Design review of the part shown in the three views and the two pictorial views. Dimensions are in mm from the part's minimum x, y and z. Give positions to 0.01 mm unless a question says otherwise; leave off trailing zeros. Loops run counter-clockwise (first coordinate to the right, second up) from the corner with the lowest first, then second, coordinate; pieces in that order, holes last. Notation, with made-up numbers: (25.5, -15) - (67.5, -15) arc R5 cw to (67.5, -9) - close; hole circle Ø10 at (-4.5, -11.75). An arc over 180 degrees is marked (long way). Use CSV: the item, a comma, the result in double quotes. Start each with the question number.
1. Take a section at C-C on z = 24.5. Give the boundary of the cut face in (x, y), plus the area to 3 significant figures.
2. Mouldability with a two-part tool opening along Y and no side actions: class the marked faces 1, 2 and 3 as pulls with the +Y half, pulls with the -Y half, needs draft (parallel to the pull), parting line crosses it, or undercut.
3. Take a section at D-D on x = 93. Give the boundary of the cut face in (y, z), plus the area to 3 significant figures.
4. Wall thickness on line 1 (Y direction, x = 10, z = 4.25); line 2 (Y direction, x = 75, z = 16.5); line 3 (Z direction, x = 90, y = 7.5): over which ranges is each line inside the solid? List them lowest first.
5. Take a section at B-B on x = 75. Give the boundary of the cut face in (y, z), plus the area to 3 significant figures.
6. Take a section at A-A on x = 140. Give the boundary of the cut face in (y, z).
7. For pin 1 (6 mm diameter, centred on y = 20, z = 22.5, fed in from +X); pin 2 (5 mm diameter, centred on x = 130, y = 14, fed in from +Z); pin 3 (4 mm diameter, centred on y = 12.5, z = 41.5, fed in from +X); pin 4 (5 mm diameter, centred on x = 38.5, y = 11.5, fed in from -Z), all flat-tipped, find the tip position at first contact; note any pin that passes through.
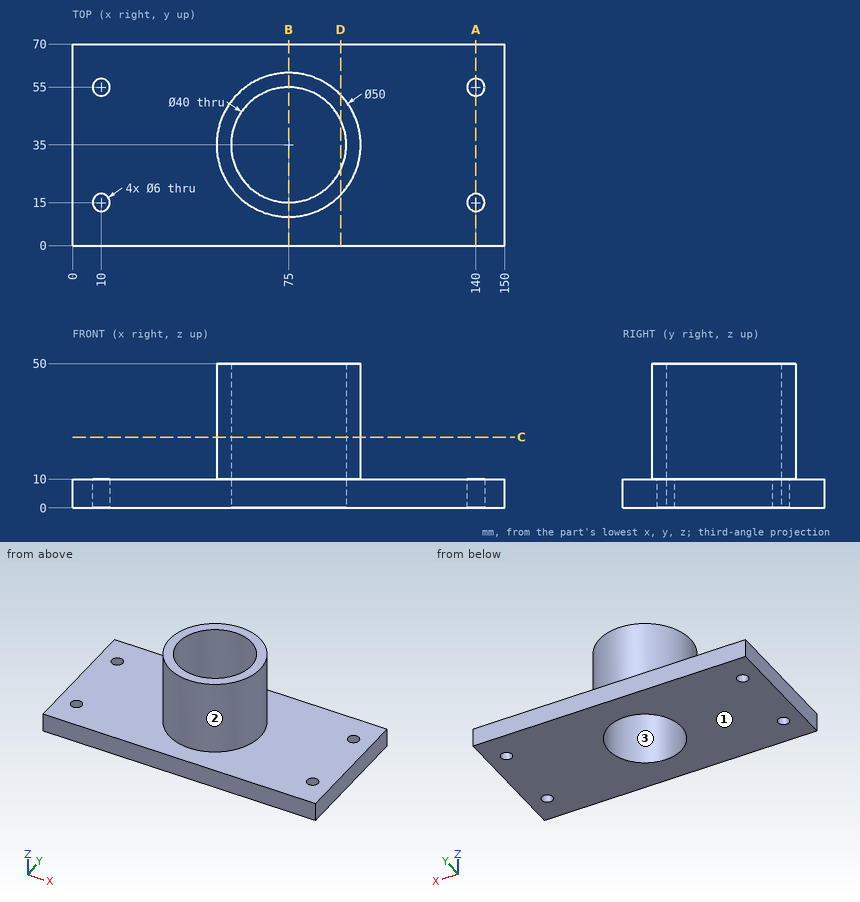
Check result:
1,outline,"circle Ø50 at (75, 35); hole circle Ø40 at (75, 35)"
1,area,"707 mm²"
2,face 1,"needs draft"
2,face 2,"parting line crosses it"
2,face 3,"undercut"
3,outline,"(0, 0) - (26.28, 0) - (26.28, 50) - (17.65, 50) - (17.65, 10) - (0, 10) - close; (43.72, 0) - (70, 0) - (70, 10) - (52.35, 10) - (52.35, 50) - (43.72, 50) - close"
3,area,"1,220 mm²"
4,line 1,"y = 0 to 12, 18 to 52, 58 to 70"
4,line 2,"y = 10 to 15, 55 to 60"
4,line 3,"z = 0 to 10"
5,outline,"(0, 0) - (15, 0) - (15, 50) - (10, 50) - (10, 10) - (0, 10) - close; (55, 0) - (70, 0) - (70, 10) - (60, 10) - (60, 50) - (55, 50) - close"
5,area,"700 mm²"
6,outline,"(0, 0) - (12, 0) - (12, 10) - (0, 10) - close; (18, 0) - (52, 0) - (52, 10) - (18, 10) - close; (58, 0) - (70, 0) - (70, 10) - (58, 10) - close"
7,pin 1,"stops at x = 96.93"
7,pin 2,"stops at z = 10"
7,pin 3,"stops at x = 89.31"
7,pin 4,"stops at z = 0"
